Autodesk Inventor part; units mm, degrees
ref_plane "YZ Plane" through (0, 0, 0) normal (1, 0, 0) x (0, 1, 0)
ref_plane "XZ Plane" through (0, 0, 0) normal (0, 1, 0) x (-1, 0, 0)
ref_plane "XY Plane" through (0, 0, 0) normal (0, 0, 1) x (1, 0, 0)
sketch "Boceto1" plane through (0, 0, 0) normal (0, 1, 0) x (-1, 0, 0)
  circle A0 centre (28.5, 0) radius 1.5
  circle A1 centre (28.5, -8) radius 1.5
  circle A2 centre (28.5, 8) radius 1.5
  circle A3 centre (36.5, 0) radius 1.5
  circle A4 centre (20.5, 0) radius 1.5
  circle A5 centre (28.5, 0) radius 47.5
  line L0 (57, 33) -> (43, 33)
  line L1 (43, 33) -> (43, 30)
  line L2 (35.5, 30) -> (35.5, 33)
  line L3 (35.5, 33) -> (21.5, 33)
  line L4 (21.5, 33) -> (21.5, 30)
  line L5 (14, 30) -> (14, 33)
  line L6 (14, 33) -> (0, 33)
  line L7 (43, 30) -> (57, 30)
  line L8 (21.5, 30) -> (35.5, 30)
  line L9 (14, 30) -> (0, 30)
  line L10 (0, 30) -> (0, 33)
  line L11 (57, 33) -> (57, 30)
  line L12 (35.5, -30) -> (35.5, -33)
  line L13 (21.5, -30) -> (35.5, -30)
  line L14 (35.5, -33) -> (21.5, -33)
  line L15 (21.5, -33) -> (21.5, -30)
  line L16 (57, -33) -> (43, -33)
  line L17 (43, -33) -> (43, -30)
  line L18 (43, -30) -> (57, -30)
  line L19 (14, -30) -> (14, -33)
  line L20 (14, -30) -> (0, -30)
  line L21 (14, -33) -> (0, -33)
  line L22 (0, -30) -> (0, -33)
  line L23 (57, -33) -> (57, -30)
extrude "Extrusión1" add sketch "Boceto1" along normal blind 3
sketch "Boceto2" plane through (-28.5, 0, 0) normal (0, -1, 0) x (1, 0, 0)
  circle A0 centre (0, 0) radius 3.5
  point P0 (28.5, 0)
  dimension "d23" = 7
extrude "Extrusión2" cut sketch "Boceto2" against normal blind 10
sketch "Boceto3" plane through (-28.5, 0, 0) normal (0, -1, 0) x (1, 0, 0)
  circle A0 centre (0, 0) radius 4.5
  point P0 (28.5, 0)
  dimension "d26" = 9
extrude "Extrusión3" cut sketch "Boceto3" against normal blind 10
sketch "Boceto4" plane through (-28.5, 0, 0) normal (0, -1, 0) x (1, 0, 0)
  circle A0 centre (0, 0) radius 4.5
  arc A1 (-38.8091, 27.388) -> (38.8091, 27.388) centre (0, 0) ccw
  line L0 (-28.5, 30) -> (-28.5, 33)
  line L1 (-28.5, 30) -> (-28.5, 33)
  line L2 (-28.5, 33) -> (28.5, 33)
  line L3 (28.5, 33) -> (28.5, 30)
  line L4 (-14.5, 30) -> (-28.5, 30)
  line L5 (28.5, 30) -> (-28.5, 30)
  line L6 (-28.5, 33) -> (-31.5138, 33)
  line L7 (-31.5138, 33) -> (-31.5138, 30)
  line L8 (-31.5138, 30) -> (-28.5, 30)
  circle A2 centre (0, 0) radius 47.5
  line L9 (38.8091, 27.388) -> (-38.8091, 27.388)
  point P0 (28.5, 0)
extrude "Extrusión4" cut sketch "Boceto4" against normal blind 10 contours L9 A1
sketch "Boceto5" plane through (0, 0, 0) normal (0, -1, 0) x (1, 0, 0)
  arc A0 (10.3091, 27.388) -> (-67.3091, 27.388) centre (-28.5, 0) ccw
  arc A1 (10.3091, 27.388) -> (-67.3091, 27.388) centre (-28.5, 0) ccw
  line L0 (-57, 19.347) -> (-43, 19.347)
  line L1 (0, 19.347) -> (-14, 19.347)
  line L2 (-14, 19.347) -> (-14, 16.347)
  line L3 (-21.5, 16.347) -> (-35.5, 16.347)
  line L4 (-43, 16.347) -> (-57, 16.347)
  line L5 (-57, 19.347) -> (-57, 16.347)
  line L6 (-43, 19.347) -> (-43, 16.347)
  line L7 (-35.5, 19.347) -> (-35.5, 16.347)
  line L8 (-21.5, 19.347) -> (-21.5, 16.347)
  line L9 (-14, 16.347) -> (0, 16.347)
  line L10 (0, 19.347) -> (0, 16.347)
  line L11 (-35.5, 19.347) -> (-21.5, 19.347)
  point P0 (0, 0)
  point P1 (-57, 30)
  point P2 (-21.5, 30)
  point P3 (0, 30)
extrude "Extrusión5" add sketch "Boceto5" against normal blind 3
sketch "Boceto6" plane through (0, 0, 0) normal (0, -1, 0) x (1, 0, 0)
  arc A0 (10.3091, 27.388) -> (-67.3091, 27.388) centre (-28.5, 0) ccw
  arc A1 (10.3091, 27.388) -> (-67.3091, 27.388) centre (-28.5, 0) ccw
  line L0 (-67.3091, 27.388) -> (10.3091, 27.388)
  point P0 (0, 0)
extrude "Extrusión6" cut sketch "Boceto6" against normal blind 3
sketch "Boceto7" plane through (0, 0, 0) normal (0, -1, 0) x (1, 0, 0)
  line L0 (-57, 19.347) -> (-43, 19.347)
  line L1 (-57, 19.347) -> (-62, 19.347)
  line L2 (-62, 19.347) -> (-62, 16.347)
  line L3 (-62, 16.347) -> (5, 16.347)
  line L4 (5, 16.347) -> (5, 19.347)
  line L5 (5, 19.347) -> (-62, 19.347)
  point P0 (0, 0)
  dimension "d36" = 5
  dimension "d37" = 67
extrude "Extrusión7" add sketch "Boceto7" along normal blind 29.5
sketch "Boceto8" plane through (0, -29.5, 0) normal (0, -1, 0) x (1, 0, 0)
  line L0 (-57, 19.347) -> (-43, 19.347)
  line L1 (-43, 16.347) -> (-57, 16.347)
  line L2 (-57, 19.347) -> (-57, 16.347)
  line L3 (-57, 16.347) -> (-43, 16.347)
  line L4 (-43, 19.347) -> (-43, 16.347)
  line L5 (-43, 16.347) -> (-43, 19.347)
  line L6 (-43, 19.347) -> (-57, 19.347)
  line L7 (-35.5, 19.347) -> (-21.5, 19.347)
  line L8 (-35.5, 19.347) -> (-35.5, 16.347)
  line L9 (-62, 16.347) -> (5, 16.347)
  line L10 (-21.5, 19.347) -> (-21.5, 16.347)
  line L11 (-35.5, 16.347) -> (-21.5, 16.347)
  line L12 (-21.5, 16.347) -> (-21.5, 19.347)
  line L13 (-21.5, 19.347) -> (-35.5, 19.347)
  line L14 (-14, 19.347) -> (0, 19.347)
  line L15 (-14, 19.347) -> (0, 19.347)
  line L16 (0, 19.347) -> (0, 16.347)
  line L17 (0, 16.347) -> (-14, 16.347)
  line L18 (-14, 16.347) -> (-14, 19.347)
  line L19 (-14, 16.347) -> (-14, 19.347)
  point P0 (0, 0)
extrude "Extrusión8" add sketch "Boceto8" along normal blind 3
properties part number "base4"
Geometry: final body of the model. Coordinates: model frame, mm. A direction names the side the tool comes from. Round coordinates to 2 decimals unless told otherwise and drop trailing zeros. Order: outer loops, then holes, each group sorted by start corner. A loop starts at its lowest first (then second) coordinate and runs counter-clockwise, first axis right, second up. Notation, with made-up numbers: (-22, -6.5) -> (-2, -6.5) arc R28 cw to (-2, 24.5) -> close; hole circle Ø1 at (15, 14.25). An arc over 180 degrees is marked (long way). Use one line per item in the form item = value.
(1) First-contact query: pin 1 Ø1.5 at (x, z) = (-17.5, 18) entering from +Y; pin 2 Ø0.9 at (y, z) = (-30.5, 17.5) entering from +X; pin 3 Ø0.9 at (y, z) = (1.5, 17.5) entering from -X. Flat tips, straight axial feed; report the tip coordinate or a pass-through.
Results list:
pin_1 = 0
pin_2 = 0
pin_3 = -57
(2) Section B-B on x = -19. Return loops of the section in (y, z).
Results list:
outline = (-29.5, 16.35) -> (0, 16.35) -> (0, 19.35) -> (-29.5, 19.35) -> close
(3) Ray query, probe 1 along X at (y, z) = (1, 18.15); probe 2 along Y at (x, z) = (-57.5, 18.5). Return the intervals inside material, ascending. Write a range as [from, to].
Results list:
probe_1 = [-57, -43], [-35.5, -21.5], [-14, 0]
probe_2 = [-29.5, 0]
(4) Section A-A on z = 18. Return loops of the section in (x, y).
Results list:
outline = (-62, -29.5) -> (-57, -29.5) -> (-57, -32.5) -> (-43, -32.5) -> (-43, -29.5) -> (-35.5, -29.5) -> (-35.5, -32.5) -> (-21.5, -32.5) -> (-21.5, -29.5) -> (-14, -29.5) -> (-14, -32.5) -> (0, -32.5) -> (0, -29.5) -> (5, -29.5) -> (5, 0) -> (0, 0) -> (0, 3) -> (-14, 3) -> (-14, 0) -> (-21.5, 0) -> (-21.5, 3) -> (-35.5, 3) -> (-35.5, 0) -> (-43, 0) -> (-43, 3) -> (-57, 3) -> (-57, 0) -> (-62, 0) -> close
(5) Draft query along X for faces 1 (the face through (-18, 0, 18)), 2 (the face through (-14, 1, 18)), 3 (the face through (-57, -31, 18)), 4 (the face through (-29, -32.5, 18)). Return one class per face: pulls with the +X half, pulls with the -X half, needs draft (parallel to the pull), parting line crosses it, or undercut.
Results list:
face_1 = undercut
face_2 = undercut
face_3 = pulls with the -X half
face_4 = needs draft
(6) Access query for faces 5 (the face through (-21.5, 1, 18)), 6 (the face through (0, 1, 18)), 7 (the face through (-14, -31, 18)). Directions: +Z, -Z, +X, -X, +Y, -Y. A direction counts if a zero-diameter tool reaches every point of the face in a straight line with its end or side. Return the directions, or none.
Results list:
face_5 = +Z, -Z, +Y
face_6 = +Z, -Z, +X, +Y
face_7 = +Z, -Z, -Y
